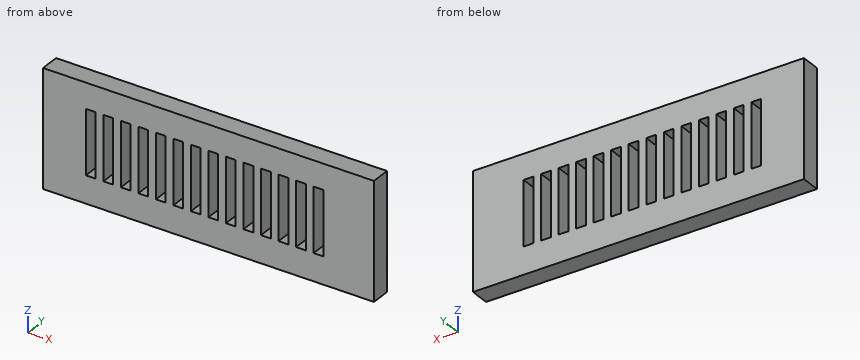
from build123d import *

# Parameters (mm, degrees)
SKETCH1_W           = 85
SKETCH1_H           = 30
BOSS_EXTRUDE1_DEPTH = 5
SKETCH2_W           = 2.5
SKETCH2_H           = 16.5
CUT_EXTRUDE1_DEPTH  = 5


with BuildPart() as part:
    # Sketch1 → Boss-Extrude1 (new body)
    with BuildSketch(Plane(origin=(0, 0, 0), x_dir=(1, 0, 0), z_dir=(0, 1, 0))):
        with Locations((42.5, 15)):
            Rectangle(SKETCH1_W, SKETCH1_H)
    extrude(amount=BOSS_EXTRUDE1_DEPTH)

    # Sketch2 → Cut-Extrude1 (cut)
    with BuildSketch(Plane(origin=(0, 5, 0), x_dir=(1, 0, 0), z_dir=(0, 1, 0))):
        with Locations((12.25, 14.75)):
            Rectangle(SKETCH2_W, SKETCH2_H)
        with Locations((16.75, 14.75)):
            Rectangle(SKETCH2_W, SKETCH2_H)
        with Locations((21.25, 14.75)):
            Rectangle(SKETCH2_W, SKETCH2_H)
        with Locations((25.75, 14.75)):
            Rectangle(SKETCH2_W, SKETCH2_H)
        with Locations((30.25, 14.75)):
            Rectangle(SKETCH2_W, SKETCH2_H)
        with Locations((34.75, 14.75)):
            Rectangle(SKETCH2_W, SKETCH2_H)
        with Locations((39.25, 14.75)):
            Rectangle(SKETCH2_W, SKETCH2_H)
        with Locations((43.75, 14.75)):
            Rectangle(SKETCH2_W, SKETCH2_H)
        with Locations((48.25, 14.75)):
            Rectangle(SKETCH2_W, SKETCH2_H)
        with Locations((52.75, 14.75)):
            Rectangle(SKETCH2_W, SKETCH2_H)
        with Locations((57.25, 14.75)):
            Rectangle(SKETCH2_W, SKETCH2_H)
        with Locations((61.75, 14.75)):
            Rectangle(SKETCH2_W, SKETCH2_H)
        with Locations((66.25, 14.75)):
            Rectangle(SKETCH2_W, SKETCH2_H)
        with Locations((70.75, 14.75)):
            Rectangle(SKETCH2_W, SKETCH2_H)
    extrude(amount=-CUT_EXTRUDE1_DEPTH, mode=Mode.SUBTRACT)


solid = part.part
For this review, take the finished solid that the model builds, in its own axes (mm). Give positions to 0.01 mm unless a question says otherwise; leave off trailing zeros. Loops run counter-clockwise (first coordinate to the right, second up) from the corner with the lowest first, then second, coordinate; pieces in that order, holes last. Notation, with made-up numbers: (56, 8.5) -> (63, 8.5) arc R23 ccw to (63, 37.5) -> close; hole circle Ø7 at (39, 83.25). An arc over 180 degrees is marked (long way). One line per question, with ' | ' between items.
1) We need section B-B (y = 2.3). Give the number of separate pieces and of enclosed holes in the cut face, plus the area to 3 significant figures.
Resolved:
separate pieces: 1 | enclosed holes: 14 | area: 1,970 mm2
2) To check wall thickness, follow probe 1 along Z at (x, y) = (31, 0.6). State the ranges of the line that lie inside material, in increasing order.
Resolved:
probe 1: z = -30 to -23, -6.5 to 0
3) We need section A-A (x = 44). Write out the cut boundary in (y, z).
Resolved:
outline: (0, -30) -> (5, -30) -> (5, -23) -> (0, -23) -> close; (0, -6.5) -> (5, -6.5) -> (5, 0) -> (0, 0) -> close
4) Insertion check: pin 1 Ø1 at (x, z) = (43, -3) entering from -Y. The pin has a flat end and moves straight along its axis. Give the tip position at first contact, or say it passes through.
Resolved:
pin 1: stops at y = 0
